```python
from build123d import *

# Parameters (mm, degrees)
SKICA1_W                = 56
SKICA1_H                = 120
SKICA1_R                = 1.5
P_IDAT_VYSUNUT_M1_DEPTH = 3
SKICA2_W                = 46
SKICA2_H                = 110
SKICA2_W_2              = 43
SKICA2_H_2              = 107
P_IDAT_VYSUNUT_M2_DEPTH = 6


with BuildPart() as part:
    # Skica1 → Přidat vysunutím1 (new body)
    with BuildSketch(Plane.XY):
        with Locations((-86, 47)):
            Rectangle(SKICA1_W, SKICA1_H)
        with Locations((-60.5, -10.5)):
            Circle(SKICA1_R, mode=Mode.SUBTRACT)
        with Locations((-111.5, -10.5)):
            Circle(SKICA1_R, mode=Mode.SUBTRACT)
        with Locations((-111.5, 27.75)):
            Circle(SKICA1_R, mode=Mode.SUBTRACT)
        with Locations((-111.5, 66)):
            Circle(SKICA1_R, mode=Mode.SUBTRACT)
        with Locations((-111.5, 104.25)):
            Circle(SKICA1_R, mode=Mode.SUBTRACT)
        with Locations((-60.5, 27.75)):
            Circle(SKICA1_R, mode=Mode.SUBTRACT)
        with Locations((-60.5, 66)):
            Circle(SKICA1_R, mode=Mode.SUBTRACT)
        with Locations((-60.5, 104.25)):
            Circle(SKICA1_R, mode=Mode.SUBTRACT)
    extrude(amount=P_IDAT_VYSUNUT_M1_DEPTH)

    # Skica2 → Přidat vysunutím2 (add)
    with BuildSketch(Plane.XY.offset(3)):
        with Locations((-86, 47)):
            Rectangle(SKICA2_W, SKICA2_H)
        with Locations((-86, 47)):
            Rectangle(SKICA2_W_2, SKICA2_H_2, mode=Mode.SUBTRACT)
    extrude(amount=-P_IDAT_VYSUNUT_M2_DEPTH)


solid = part.part
```
Here's how the part is built. I have some questions about the finished solid (model axes, mm). A direction names the side the tool comes from. Give positions to 0.01 mm unless a question says otherwise; leave off trailing zeros. Order: outer loops, then holes, each group sorted by start corner. A loop starts at its lowest first (then second) coordinate and runs counter-clockwise, first axis right, second up. Notation, with made-up numbers: (28.5, 76.5) - (46.5, 76.5) arc R30 ccw to (46.5, 107.5) - close; hole circle Ø3 at (43.5, 52.25). An arc over 180 degrees is marked (long way). Answer as a JSON object with one key per item and string values. Group by question number.
Item 1: If we section it at C-C on z = -1.05: Please give me the cut outline in (x, y).
Item 2: If we section it at A-A on x = -60.5: Please give me the cut outline in (y, z).
Item 3: Which directions (+Z, -Z, +X, -X, +Y, -Y) give clear straight access to the entire face, cutting with the end or side of a thin tool? Please do faces 5 (the flat face through (-86, -8, -1)), 6 (the flat face through (-107.5, 46, -1)), 7 (the flat face through (-86, 102, -1)).
Item 4: If we mould it in two halves opening along Y, with no side actions, what happens to faces 1 (the flat face through (-109, 46, -1)), 2 (the flat face through (-86, 107, 1)), 3 (the flat face through (-86, -13, 1)), 4 (the cylindrical face through (-59, 66, 1))? For each: pulls with the +Y half, pulls with the -Y half, needs draft (parallel to the pull), parting line crosses it, or undercut.
Item 5: Please list where these lines run through material, in increasing order: probe 1 along Y at (x, z) = (-60.5, 2.35); probe 2 along X at (y, z) = (69, -0.8); probe 3 along Y at (x, z) = (-73, -0.75).
Item 6: If we section it at D-D on x = -88.5: Please give me the cut outline in (y, z), and give its area (3 significant figures).
Item 7: For P1, Ø1.8, axis at x = -111.5, y = 104.25, coming from the -Z side; P2, Ø0.9, axis at x = -87, z = -1.5, coming from the -Y side; P3, Ø1.5, axis at x = -85, z = -1.5, coming from the +Y side; P4, Ø1.5, axis at y = 20.5, z = -1, coming from the -X side, each with a flat end and sliding along its axis, tell me the tip position at first contact or that it passes through.
Item 8: If we section it at B-B on y = 104.25: Please give me the cut outline in (x, z).
Result set:
{
 "1": {"outline": "(-109, -8) - (-63, -8) - (-63, 102) - (-109, 102) - close; hole (-107.5, -6.5) - (-64.5, -6.5) - (-64.5, 100.5) - (-107.5, 100.5) - close"},
 "2": {"outline": "(-13, 0) - (-12, 0) - (-12, 3) - (-13, 3) - close; (-9, 0) - (26.25, 0) - (26.25, 3) - (-9, 3) - close; (29.25, 0) - (64.5, 0) - (64.5, 3) - (29.25, 3) - close; (67.5, 0) - (102.75, 0) - (102.75, 3) - (67.5, 3) - close; (105.75, 0) - (107, 0) - (107, 3) - (105.75, 3) - close"},
 "3": {"face 5": "-Z, +X, -X, -Y", "face 6": "-Z", "face 7": "-Z, +X, -X, +Y"},
 "4": {"face 1": "needs draft", "face 2": "pulls with the +Y half", "face 3": "pulls with the -Y half", "face 4": "undercut"},
 "5": {"probe 1": "-13 to -12, -9 to 26.25, 29.25 to 64.5, 67.5 to 102.75, 105.75 to 107", "probe 2": "-109 to -107.5, -64.5 to -63", "probe 3": "-8 to -6.5, 100.5 to 102"},
 "6": {"outline": "(-13, 0) - (-8, 0) - (-8, -3) - (-6.5, -3) - (-6.5, 0) - (100.5, 0) - (100.5, -3) - (102, -3) - (102, 0) - (107, 0) - (107, 3) - (-13, 3) - close", "area": "369 mm²"},
 "7": {"P1": "through", "P2": "y = -8", "P3": "y = 102", "P4": "x = -109"},
 "8": {"outline": "(-114, 0) - (-113, 0) - (-113, 3) - (-114, 3) - close; (-110, 0) - (-62, 0) - (-62, 3) - (-110, 3) - close; (-59, 0) - (-58, 0) - (-58, 3) - (-59, 3) - close"}
}
